from build123d import *

# Parameters (mm, degrees)
ESQUISSE1_W                  = 144
ESQUISSE1_H                  = 337
BOSS_EXTRU_1_DEPTH           = 3
ESQUISSE2_R                  = 1.5
ENL_V_MAT_EXTRU_1_DEPTH      = 367.488744711
CHANFREIN1_SIZE              = 49
ENL_V_MAT_EXTRU_2_DEPTH      = 367.488744711
ENL_V_MAT_EXTRU_2_DEPTH_BACK = 367.488744711
ESQUISSE3_W                  = 10
ESQUISSE3_H                  = 35
ESQUISSE4_W                  = 22
ESQUISSE4_H                  = 13
ENL_V_MAT_EXTRU_3_DEPTH      = 367.488744711
ENL_V_MAT_EXTRU_4_DEPTH      = 367.488744711
ENL_V_MAT_EXTRU_7_DEPTH      = 367.488744711
BOSS_EXTRU_3_DEPTH           = 3
CONG_4_R                     = 3


with BuildPart() as part:
    # Esquisse1 → Boss.-Extru.1 (new body)
    with BuildSketch(Plane.XY):
        with Locations((72, 168.5)):
            Rectangle(ESQUISSE1_W, ESQUISSE1_H)
    extrude(amount=BOSS_EXTRU_1_DEPTH)

    # Esquisse2 → Enlèv. mat.-Extru.1 (cut, through all)
    with BuildSketch(Plane.XY.offset(3)):
        with Locations((16, 22)):
            Circle(ESQUISSE2_R)
        with Locations((12.5, 234)):
            Circle(ESQUISSE2_R)
        with Locations((12.5, 134)):
            Circle(ESQUISSE2_R)
        with Locations((68, 315.5)):
            Circle(ESQUISSE2_R)
        with Locations((128, 315.5)):
            Circle(ESQUISSE2_R)
        with Locations((117, 22)):
            Circle(ESQUISSE2_R)
    extrude(amount=-ENL_V_MAT_EXTRU_1_DEPTH, mode=Mode.SUBTRACT)

    # Chanfrein1
    chanfrein1_edges = [part.edges().sort_by_distance(p)[0] for p in [
        (0, 337, 1.5),
    ]]
    chamfer(chanfrein1_edges, length=CHANFREIN1_SIZE)

    # Esquisse3 → Enlèv. mat.-Extru.2 (cut, two sides: drawn at the far end of the back side and taken through both)
    with BuildSketch(Plane.XY.offset(3).offset(-ENL_V_MAT_EXTRU_2_DEPTH_BACK)):
        with Locations((139, 17.5)):
            Rectangle(ESQUISSE3_W, ESQUISSE3_H)
    extrude(amount=ENL_V_MAT_EXTRU_2_DEPTH + ENL_V_MAT_EXTRU_2_DEPTH_BACK, mode=Mode.SUBTRACT)

    # Esquisse4 → Enlèv. mat.-Extru.3 (cut, through all)
    with BuildSketch(Plane.XY.offset(3)):
        with Locations((24, 57.5)):
            Rectangle(ESQUISSE4_W, ESQUISSE4_H)
    extrude(amount=-ENL_V_MAT_EXTRU_3_DEPTH, mode=Mode.SUBTRACT)

    # Esquisse5 → Enlèv. mat.-Extru.4 (cut, through all)
    with BuildSketch(Plane.XY.offset(3)):
        with BuildLine():
            Line((144, 60), (90, 60))
            Line((90, 60), (90, 190))
            ThreePointArc((90, 190), (68.473980144, 267.875312279), (144, 296.576429297))
            Line((144, 296.576429297), (144, 60))
        make_face()
    extrude(amount=-ENL_V_MAT_EXTRU_4_DEPTH, mode=Mode.SUBTRACT)

    # Esquisse9 → Enlèv. mat.-Extru.7 (cut, through all)
    with BuildSketch(Plane.XY.offset(3)):
        Polygon((94, 102), (34, 102), (34, 146), (54, 146), (54, 158), (74, 158), (74, 146), (94, 146), align=None)
    extrude(amount=-ENL_V_MAT_EXTRU_7_DEPTH, mode=Mode.SUBTRACT)

    # Esquisse10 → Boss.-Extru.3 (add)
    with BuildSketch(Plane.XY.offset(3)):
        Polygon((144, 60), (90, 60), (90, 102), (94, 102), (94, 146), (90, 146), (90, 190), (55, 190), (55, 302), (144, 302), align=None)
    extrude(amount=-BOSS_EXTRU_3_DEPTH)

    # Congé4
    cong_4_edges = [part.edges().sort_by_distance(p)[0] for p in [
        (74, 146, 1.5),
        (34, 102, 1.5),
        (34, 146, 1.5),
        (54, 146, 1.5),
        (54, 158, 1.5),
        (74, 158, 1.5),
        (94, 102, 1.5),
        (94, 146, 1.5),
        (134, 35, 1.5),
        (13, 51, 1.5),
        (13, 64, 1.5),
        (35, 64, 1.5),
        (35, 51, 1.5),
    ]]
    fillet(cong_4_edges, radius=CONG_4_R)


solid = part.part
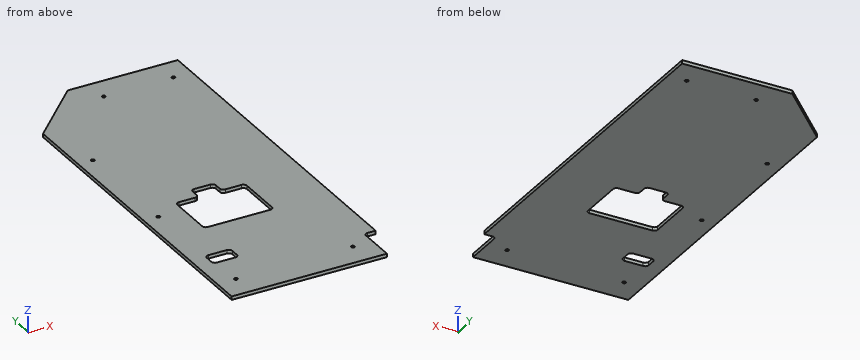
Verification items for the finished model (mm, model axes). Coordinates: 2 decimals unless noted, no trailing zeros. Write each loop counter-clockwise with the first axis right and the second up, starting at its lowest first coordinate (ties: lowest second). Pieces come first, ordered by that corner, then holes. Notation, with made-up numbers: (85, -12.75) -> (130, -12.75) arc R6 ccw to (130, -1.75) -> close; hole circle Ø7 at (29, 17.25). An arc over 180 degrees is marked (long way). One line per item, written item: value. Start each with the question number.
Q1. Cross-section at B-B on z = 1.9. State how many separate pieces and enclosed holes the cut face has, and give its area (3 significant figures).
Q2. Cross-section at A-A on y = 305. Enter the section's corners in (x, z).
Q3. Thickness scan on L1, parallel to X at y = 134, z = 2.2; L2, parallel to X at y = 234, z = 1.9; L3, parallel to Y at x = 65, z = 0.75. Record the ranges inside material, lowest first. Write a range as from..to.
Q4. Go/stop test with flat-tipped pins: P1, Ø1.5, axis at x = 23, z = 1, coming from the +Y side; P2, Ø1.5, axis at y = 12.5, z = 2, coming from the +X side. Record where each tip stops, or that it passes through.
Checked values:
1. separate pieces: 1
1. enclosed holes: 8
1. area: 43,800 mm²
2. outline: (17, 0) -> (144, 0) -> (144, 3) -> (17, 3) -> close
3. L1: x = 0..11, 14..34, 94..144
3. L2: x = 0..11, 14..144
3. L3: y = 0..102, 158..337
4. P1: stops at y = 311.75
4. P2: stops at x = 134
